Part model, mm, in its own coordinate system. A direction names the side the tool comes from. Coordinates: 2 decimals unless noted, no trailing zeros. Order: outer loops, then holes, each group sorted by start corner. A loop starts at its lowest first (then second) coordinate and runs counter-clockwise, first axis right, second up. Notation, with made-up numbers: M -25.75,-23 L -16.75,-23 A18 cw -16.75,1 Z; hole C 3,17.5 d3. An arc over 180 degrees is marked long. Answer in a Markdown table with one row per item. Add a question column.
from build123d import *

# Parameters (mm, degrees)
F0_W     = 152.4
F0_H     = 127
F1_DEPTH = 50.8
F3_DEPTH = 50.801
F5_W     = 62.23
F5_H     = 43.18
F6_DEPTH = 62.231
F7_F1_R  = 5.08
F7_F2_R  = 5.08
F7_F3_R  = 5.08
F7_F4_R  = 5.08
F7_F5_R  = 5.08
F7_F6_R  = 5.08
F7_F7_R  = 5.08
F7_F8_R  = 5.08
F7_F9_R  = 5.08
F7_F10_R = 5.08
F7_F11_R = 5.08
F7_F12_R = 5.08
F7_F13_R = 5.08
F7_F14_R = 5.08
F7_F15_R = 5.08
F7_F16_R = 5.08


# Not quite as in the source:
# - a pattern or mirror of a feature is missing from the dataset's text; its kind, count and spacing are read off the source's solid


with BuildPart() as f1:
    # F0 (on Top) → F1 (new body)
    with BuildSketch(Plane.XY):
        Rectangle(F0_W, F0_H)
    extrude(amount=F1_DEPTH)

    # F2 (on face) → F3 (cut, through all)
    with BuildSketch(Plane.XY.offset(50.8)):
        with BuildLine():
            Line((-71.12, -63.5), (71.12, -63.5))
            ThreePointArc((71.12, -63.5), (0, -25.4), (-71.12, -63.5))
        make_face()
        with BuildLine():
            ThreePointArc((-71.12, 63.5), (0, 25.4), (71.12, 63.5))
            Line((71.12, 63.5), (-71.12, 63.5))
        make_face()
    extrude(amount=-F3_DEPTH, mode=Mode.SUBTRACT)

    # F5 (on offset) → F6 (cut, through all)
    with BuildSketch(Plane.XZ.offset(1.27)):
        with Locations((-34.925, 25.4)):
            Rectangle(F5_W, F5_H)
        with Locations((34.925, 25.4)):
            Rectangle(F5_W, F5_H)
    f6 = extrude(amount=F6_DEPTH, mode=Mode.SUBTRACT)

    # F6_copies: F6 across plane
    add(f6.mirror(Plane.ZX), mode=Mode.SUBTRACT)

    # F7: fillet of radius 5.08 on 28 edges, made by hand

    # F7_f1
    f7_f1_edges = [f1.edges().sort_by_distance(p)[0] for p in [
        (34.925, -1.27, 3.81),
    ]]
    fillet(f7_f1_edges, radius=F7_F1_R)

    # F7_f2
    f7_f2_edges = [f1.edges().sort_by_distance(p)[0] for p in [
        (66.04, -31.4933212262, 3.81),
    ]]
    fillet(f7_f2_edges, radius=F7_F2_R)

    # F7_f3
    f7_f3_edges = [f1.edges().sort_by_distance(p)[0] for p in [
        (3.81, -15.9175013231, 3.81),
    ]]
    fillet(f7_f3_edges, radius=F7_F3_R)

    # F7_f4
    f7_f4_edges = [f1.edges().sort_by_distance(p)[0] for p in [
        (3.81, -15.9175013231, 46.99),
    ]]
    fillet(f7_f4_edges, radius=F7_F4_R)

    # F7_f5
    f7_f5_edges = [f1.edges().sort_by_distance(p)[0] for p in [
        (-34.925, -1.27, 3.81),
    ]]
    fillet(f7_f5_edges, radius=F7_F5_R)

    # F7_f6
    f7_f6_edges = [f1.edges().sort_by_distance(p)[0] for p in [
        (-3.81, -15.9175013231, 3.81),
    ]]
    fillet(f7_f6_edges, radius=F7_F6_R)

    # F7_f7
    f7_f7_edges = [f1.edges().sort_by_distance(p)[0] for p in [
        (-66.04, -31.4933212262, 3.81),
    ]]
    fillet(f7_f7_edges, radius=F7_F7_R)

    # F7_f8
    f7_f8_edges = [f1.edges().sort_by_distance(p)[0] for p in [
        (-66.04, -31.4933212262, 46.99),
    ]]
    fillet(f7_f8_edges, radius=F7_F8_R)

    # F7_f9
    f7_f9_edges = [f1.edges().sort_by_distance(p)[0] for p in [
        (-3.81, 1.27, 25.4),
    ]]
    fillet(f7_f9_edges, radius=F7_F9_R)

    # F7_f10
    f7_f10_edges = [f1.edges().sort_by_distance(p)[0] for p in [
        (-37.465, 1.27, 46.99),
    ]]
    fillet(f7_f10_edges, radius=F7_F10_R)

    # F7_f11
    f7_f11_edges = [f1.edges().sort_by_distance(p)[0] for p in [
        (-66.04, 31.4933212262, 46.99),
    ]]
    fillet(f7_f11_edges, radius=F7_F11_R)

    # F7_f12
    f7_f12_edges = [f1.edges().sort_by_distance(p)[0] for p in [
        (-66.04, 31.4933212262, 3.81),
    ]]
    fillet(f7_f12_edges, radius=F7_F12_R)

    # F7_f13
    f7_f13_edges = [f1.edges().sort_by_distance(p)[0] for p in [
        (34.925, 1.27, 3.81),
    ]]
    fillet(f7_f13_edges, radius=F7_F13_R)

    # F7_f14
    f7_f14_edges = [f1.edges().sort_by_distance(p)[0] for p in [
        (66.04, 31.4933212262, 3.81),
    ]]
    fillet(f7_f14_edges, radius=F7_F14_R)

    # F7_f15
    f7_f15_edges = [f1.edges().sort_by_distance(p)[0] for p in [
        (66.04, 31.4933212262, 46.99),
    ]]
    fillet(f7_f15_edges, radius=F7_F15_R)

    # F7_f16
    f7_f16_edges = [f1.edges().sort_by_distance(p)[0] for p in [
        (3.81, 1.27, 25.4),
    ]]
    fillet(f7_f16_edges, radius=F7_F16_R)


solid = f1.part
(1) 3-axis set-ups, long thin cutter, end or side, ignore diameter. For faces 1 (the cylindrical face through (1.18, -25.41, 25.76)), 2 (the cylindrical face through (-64.591, -2.798, 25.169)), 3 (the flat face through (-41, 23, 46.99)): which of +Z, -Z, +X, -X, +Y, -Y reach the whole face in a straight line?
(2) Wall check: line 1 (X direction, y = -20.5, z = 13); line 2 (X direction, y = -45, z = 28); line 3 (X direction, y = -24, z = 46). Give the ranges that are in metal, low to high.
(3) Slice it at D-D (x = -43). List the corners of the cut face in (y, z), and give its area (3 significant figures).
(4) Slice it at B-B (y = 44). List the corners of the cut face in (x, z), and give its area (3 significant figures).
(5) Pull direction X, two halves, no side cores. Call faces 4 (the flat face through (76.2, -1, 25)), 5 (the flat face through (-1, 1, 0)), 6 (the flat face through (3.81, -16, 25)), 7 (the cylindrical face through (5.338, -16.244, 45.541)): pulls with the +X half, pulls with the -X half, needs draft (parallel to the pull), parting line crosses it, or undercut.
(6) Drop flat-ended pins along their axis: P1, Ø6, axis at x = -56.5, z = 20, coming from the +Y side; P2, Ø12, axis at x = -3, z = 32.5, coming from the +Y side (3 decimals). Give the stop position or say it passes through.
(7) Slice it at C-C (y = -12.5). List the corners of the cut face in (x, z).
Computed:
| question | item | result |
|---|---|---|
| 1 | face 1 | +Z, -Z, -Y |
| 1 | face 2 | -Y |
| 1 | face 3 | +Y |
| 2 | line 1 | x = -76.2 to -66.04, -3.81 to 3.81, 66.04 to 76.2 |
| 2 | line 2 | x = -76.2 to -66.04, 66.04 to 76.2 |
| 2 | line 3 | x = -76.2 to -63.97, -5.88 to 5.88, 63.97 to 76.2 |
| 3 | outline | M -37.01,0 L 37.01,0 L 37.01,3.81 L 6.35,3.81 A5.08 cw 1.27,8.89 L 1.27,41.91 A5.08 cw 6.35,46.99 L 37.01,46.99 L 37.01,50.8 L -37.01,50.8 L -37.01,46.99 L -6.35,46.99 A5.08 cw -1.27,41.91 L -1.27,8.89 A5.08 cw -6.35,3.81 L -37.01,3.81 Z |
| 3 | area | 696 mm^2 |
| 4 | outline | M -76.2,0 L -53.22,0 L -53.22,3.81 L -60.96,3.81 A5.08 cw -66.04,8.89 L -66.04,41.91 A5.08 cw -60.96,46.99 L -53.22,46.99 L -53.22,50.8 L -76.2,50.8 Z; M 53.22,0 L 76.2,0 L 76.2,50.8 L 53.22,50.8 L 53.22,46.99 L 60.96,46.99 A5.08 cw 66.04,41.91 L 66.04,8.89 A5.08 cw 60.96,3.81 L 53.22,3.81 Z |
| 4 | area | 1,250 mm^2 |
| 5 | face 4 | pulls with the +X half |
| 5 | face 5 | needs draft |
| 5 | face 6 | undercut |
| 5 | face 7 | undercut |
| 6 | P1 | stops at y = 1.27 |
| 6 | P2 | stops at y = 25.485 |
| 7 | outline | M -76.2,0 L 76.2,0 L 76.2,50.8 L -76.2,50.8 Z; hole M -66.04,8.89 A5.08 ccw -60.96,3.81 L -8.89,3.81 A5.08 ccw -3.81,8.89 L -3.81,41.91 A5.08 ccw -8.89,46.99 L -60.96,46.99 A5.08 ccw -66.04,41.91 Z; hole M 3.81,8.89 A5.08 ccw 8.89,3.81 L 60.96,3.81 A5.08 ccw 66.04,8.89 L 66.04,41.91 A5.08 ccw 60.96,46.99 L 8.89,46.99 A5.08 ccw 3.81,41.91 Z |
